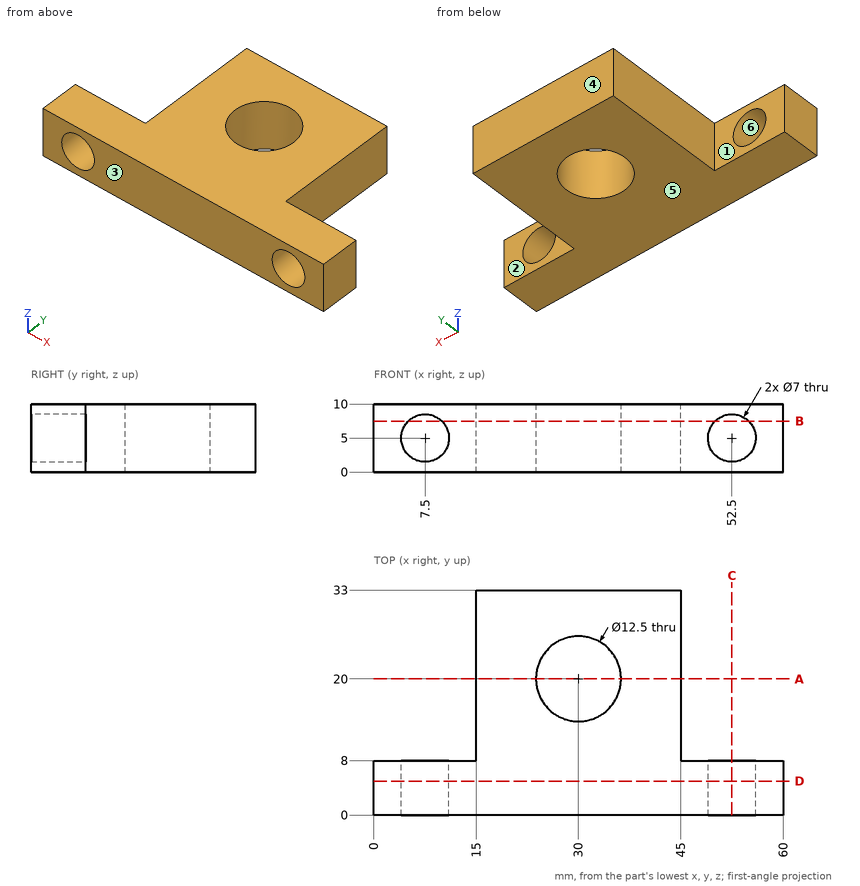
Job drawing, mm, ordinate dimensions from the low corner. One solid piece. A direction names the side the tool comes from. Give positions to 0.01 mm unless a question says otherwise; leave off trailing zeros. Order: outer loops, then holes, each group sorted by start corner. A loop starts at its lowest first (then second) coordinate and runs counter-clockwise, first axis right, second up. Notation, with made-up numbers: M 58,-32 L 74,-32 A22 ccw 74,6 Z; hole C 49.5,-20 d1. An arc over 180 degrees is marked long. Return JSON: item names as keys, results as strings.
Q1. Band-saw the part on B-B (z = 7.5). Give the cut face in (x, y).
Answer list:
{"outline": "M 0,0 L 5.05,0 L 5.05,8 L 0,8 Z; M 9.95,0 L 50.05,0 L 50.05,8 L 45,8 L 45,33 L 15,33 L 15,8 L 9.95,8 Z; M 54.95,0 L 60,0 L 60,8 L 54.95,8 Z; hole C 30,20 d12.5"}
Q2. Wall check: probe 1 along X at (y, z) = (6.25, 5); probe 2 along X at (y, z) = (6.5, 3.5); probe 3 along X at (y, z) = (13, 9.5). Give the ranges that are in metal, low to high. Write a range as from..to.
Answer list:
{"probe 1": "x = 0..4, 11..49, 56..60", "probe 2": "x = 0..4.34, 10.66..49.34, 55.66..60", "probe 3": "x = 15..45"}
Q3. Flat gauge pins, fed straight in: pin 1 (3 mm diameter, centred on y = 20.5, z = 7, fed in from -X); pin 2 (1 mm diameter, centred on x = 53.5, z = 4.5, fed in from +Y); pin 3 (5 mm diameter, centred on y = 22, z = 6.5, fed in from +X). Where does each tip first touch, or does it go through?
Answer list:
{"pin 1": "stops at x = 15", "pin 2": "passes through", "pin 3": "stops at x = 45"}
Q4. Band-saw the part on A-A (y = 20). Give the cut face in (x, z).
Answer list:
{"outline": "M 15,0 L 23.75,0 L 23.75,10 L 15,10 Z; M 36.25,0 L 45,0 L 45,10 L 36.25,10 Z"}
Q5. 3-axis set-ups, long thin cutter, end or side, ignore diameter. For the marked faces 1, 2 and 3: which of +Z, -Z, +X, -X, +Y, -Y reach the whole face in a straight line?
Answer list:
{"face 1": "+Z, -Z, -X, +Y", "face 2": "+Z, -Z, +X, +Y", "face 3": "+Z, -Z, +X, -X, -Y"}
Q6. Two-plate mould, pull along Z, no slides. Class the marked faces 4, 5 and 6: pulls with the +Z half, pulls with the -Z half, needs draft (parallel to the pull), parting line crosses it, or undercut.
Answer list:
{"face 4": "needs draft", "face 5": "pulls with the -Z half", "face 6": "undercut"}
Q7. Band-saw the part on D-D (y = 5). Give the cut face in (x, z), then the cut area to 3 significant figures.
Answer list:
{"outline": "M 0,0 L 60,0 L 60,10 L 0,10 Z; hole C 7.5,5 d7; hole C 52.5,5 d7", "area": "523 mm^2"}
Q8. Band-saw the part on C-C (x = 52.5). Give the cut face in (y, z).
Answer list:
{"outline": "M 0,0 L 8,0 L 8,1.5 L 0,1.5 Z; M 0,8.5 L 8,8.5 L 8,10 L 0,10 Z"}
